from build123d import *

# Parameters (mm, degrees)
SKETCH1_W           = 76.2
SKETCH1_H           = 88.9
SKETCH1_W_2         = 63.5
SKETCH1_H_2         = 25.4
BOSS_EXTRUDE1_DEPTH = 6.35
SKETCH2_W           = 6.35
SKETCH2_H           = 9.525
SKETCH2_W_2         = 9.525
SKETCH2_H_2         = 6.35
BOSS_EXTRUDE3_DEPTH = 6.35


with BuildPart() as part:
    # Sketch1 → Boss-Extrude1 (new body)
    with BuildSketch(Plane.XY):
        with Locations((38.1, -44.45)):
            Rectangle(SKETCH1_W, SKETCH1_H)
        with Locations((38.1, -69.85)):
            Rectangle(SKETCH1_W_2, SKETCH1_H_2, mode=Mode.SUBTRACT)
    extrude(amount=BOSS_EXTRUDE1_DEPTH)

    # Sketch2 → Boss-Extrude3 (add)
    with BuildSketch(Plane.XY.offset(6.35)):
        with Locations((-3.175, -14.2875)):
            Rectangle(SKETCH2_W, SKETCH2_H)
        with Locations((-3.175, -33.3375)):
            Rectangle(SKETCH2_W, SKETCH2_H)
        with Locations((-3.175, -52.3875)):
            Rectangle(SKETCH2_W, SKETCH2_H)
        with Locations((-3.175, -71.4375)):
            Rectangle(SKETCH2_W, SKETCH2_H)
        with Locations((4.7625, -92.075)):
            Rectangle(SKETCH2_W_2, SKETCH2_H_2)
        with Locations((23.8125, -92.075)):
            Rectangle(SKETCH2_W_2, SKETCH2_H_2)
        with Locations((79.375, -71.4375)):
            Rectangle(SKETCH2_W, SKETCH2_H)
        with Locations((79.375, -52.3875)):
            Rectangle(SKETCH2_W, SKETCH2_H)
        with Locations((79.375, -33.3375)):
            Rectangle(SKETCH2_W, SKETCH2_H)
        with Locations((79.375, -14.2875)):
            Rectangle(SKETCH2_W, SKETCH2_H)
        with Locations((42.8625, -92.075)):
            Rectangle(SKETCH2_W_2, SKETCH2_H_2)
        with Locations((61.9125, -92.075)):
            Rectangle(SKETCH2_W_2, SKETCH2_H_2)
    extrude(amount=-BOSS_EXTRUDE3_DEPTH)


solid = part.part
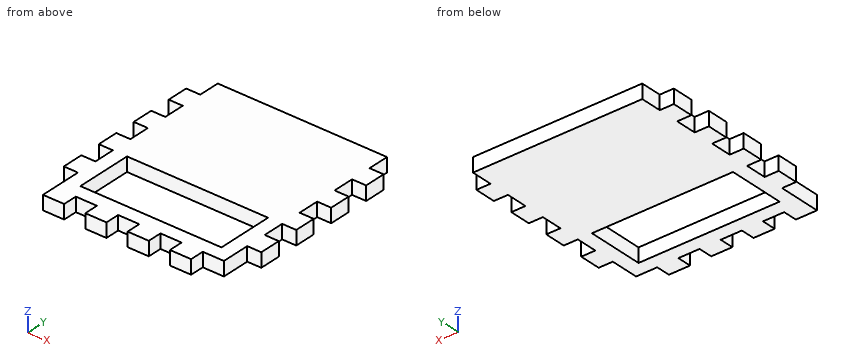
Check sheet for the modelled part. Datum: model origin and axes. Units: mm. Give positions to 0.01 mm unless a question says otherwise; leave off trailing zeros. Order: outer loops, then holes, each group sorted by start corner. A loop starts at its lowest first (then second) coordinate and runs counter-clockwise, first axis right, second up. Notation, with made-up numbers: M -34,80.25 L 15,80.25 A31 cw 15,119.25 Z; hole C 5.5,-37.5 d6. An arc over 180 degrees is marked long. Answer as CSV lines item,"result". Start each with the question number.
Item 1: Cross-section at B-B on y = -69.5. Enter the section's corners in (x, z).
Item 2: Gauge pin test, flat ends, axial feed: P1, Ø3, axis at y = -83.5, z = 4.5, coming from the +X side; P2, Ø1.9, axis at x = -3, z = 2, coming from the +Y side (3 decimals); P3, Ø3, axis at y = -93, z = 4.5, coming from the +X side (3 decimals). Record the tip position at first contact, or that the pin passes through.
Item 3: Cross-section at C-C on x = 72. Enter the section's corners in (y, z), plus the area to 3 significant figures.
Item 4: Cross-section at A-A on x = 32.5. Enter the section's corners in (y, z).
Item 5: Cross-section at D-D on y = -25.5. Enter the section's corners in (x, z), plus the area to 3 significant figures.
Item 6: Thickness scan on line 1 (Y direction, x = 76.5, z = 5) (3 decimals); line 2 (X direction, y = -90, z = 5) (3 decimals); line 3 (Y direction, x = 53, z = 4). Record the ranges inside material, lowest first. Write a range as [from, to].
Established:
1,outline,"M -6.35,0 L 6.35,0 L 6.35,6.35 L -6.35,6.35 Z; M 69.85,0 L 82.55,0 L 82.55,6.35 L 69.85,6.35 Z"
2,P1,"stops at x = 76.2"
2,P2,"stops at y = -9.525"
2,P3,"stops at x = 66.675"
3,outline,"M -88.9,0 L 0,0 L 0,6.35 L -88.9,6.35 Z"
3,area,"565 mm^2"
4,outline,"M -88.9,0 L -82.55,0 L -82.55,6.35 L -88.9,6.35 Z; M -57.15,0 L 0,0 L 0,6.35 L -57.15,6.35 Z"
5,outline,"M 0,0 L 76.2,0 L 76.2,6.35 L 0,6.35 Z"
5,area,"484 mm^2"
6,line 1,"y = [-76.2, -66.675], [-57.15, -47.625], [-38.1, -28.575], [-19.05, -9.525]"
6,line 2,"x = [0, 9.525], [19.05, 28.575], [38.1, 47.625], [57.15, 66.675]"
6,line 3,"y = [-88.9, -82.55], [-57.15, 0]"
